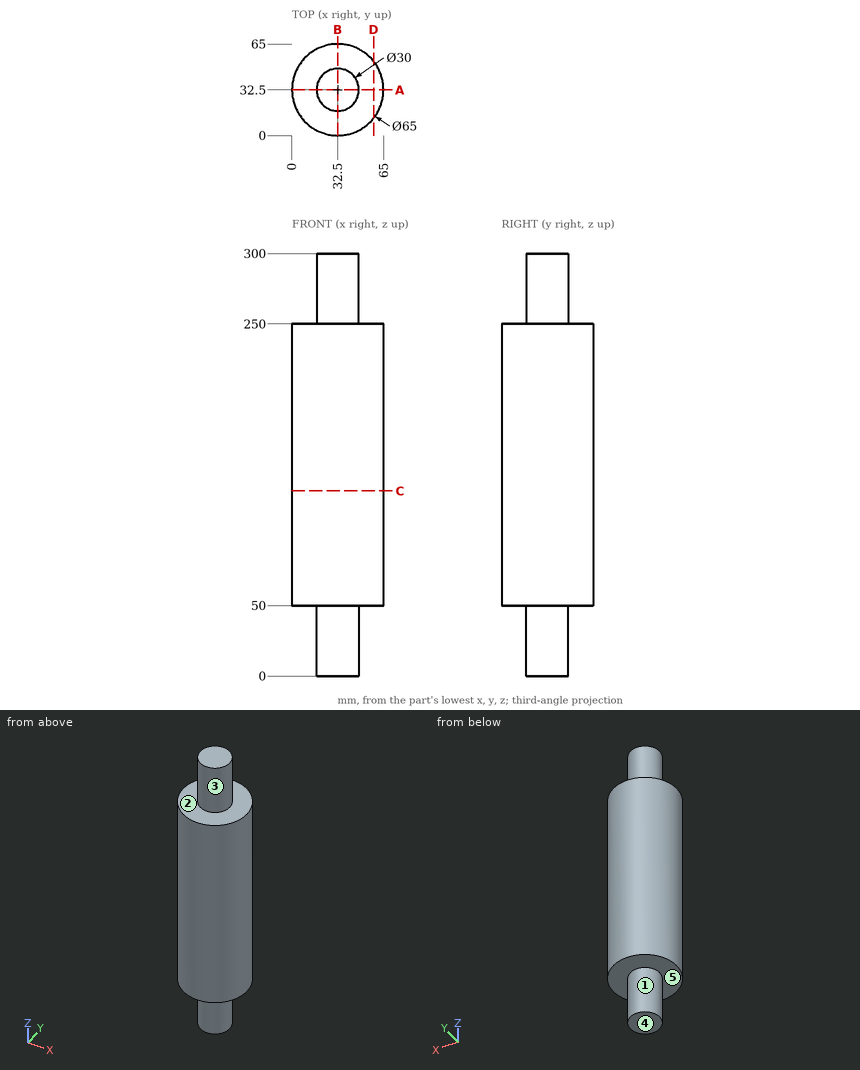
Here's the drawing with two shaded views (mm, measured from the low corner). I have some questions. A direction names the side the tool comes from. Coordinates: 2 decimals unless noted, no trailing zeros. Write each loop counter-clockwise with the first axis right and the second up, starting at its lowest first coordinate (ties: lowest second). Pieces come first, ordered by that corner, then holes.
Item 1: If we mould it in two halves opening along X, with no side actions, what happens to the marked faces 1 and 2? For each: +X half, -X half, draft (parallel to the pull), parting line (faces both ways), or undercut.
Item 2: On a 3-axis mill with a long thin cutter (end or side, diameter ignored), from which of +Z, -Z, +X, -X, +Y, -Y can I reach the whole of each face in a straight line? I mean the marked faces 3, 4 and 5. Say none if no direction works.
Item 3: If I drill on line 1 (Z direction, x = 41, y = 47); line 2 (Y direction, x = 32, z = 127); line 3 (Y direction, x = 7, z = 160), over which ranges is the centre line in solid material (lowest first)?
Item 4: I want a section at A-A on y = 32.5. Write out the boundary of the cut face in (x, z).
Item 5: I want a section at C-C on z = 131.5. Write out the boundary of the cut face in (x, y).
Item 6: I want a section at D-D on x = 58. Write out the boundary of the cut face in (y, z), and give its area (3 significant figures).
Item 7: Will these pins go through, and if not, where does the flat tip stop? pin 1 (2 mm diameter, centred on y = 15, z = 234, fed in from +X); pin 2 (6 mm diameter, centred on x = 6.5, y = 28.5, fed in from +Z); pin 3 (1.5 mm diameter, centred on x = 33, y = 56, fed in from -Z).
Findings below:
1. face 1: parting line
1. face 2: draft
2. face 3: +Z
2. face 4: -Z, +X, -X, +Y, -Y
2. face 5: -Z
3. line 1: z = 50 to 250
3. line 2: y = 0 to 65
3. line 3: y = 12.35 to 52.65
4. outline: (0, 50) - (17.5, 50) - (17.5, 0) - (47.5, 0) - (47.5, 50) - (65, 50) - (65, 250) - (47.5, 250) - (47.5, 300) - (17.5, 300) - (17.5, 250) - (0, 250) - close
5. outline: circle Ø65 at (32.5, 32.5)
6. outline: (12.35, 50) - (52.65, 50) - (52.65, 250) - (12.35, 250) - close
6. area: 8,060 mm2
7. pin 1: stops at x = 60.5
7. pin 2: stops at z = 250
7. pin 3: stops at z = 50
